Autodesk Inventor part; units mm, degrees
ref_plane "Work Plane1" through (8, 0, 0) normal (0, -0.5, -0.866) x (1, 0, 0)
ref_plane "YZ Plane" through (0, 0, 0) normal (1, 0, 0) x (0, 1, 0)
ref_plane "XZ Plane" through (0, 0, 0) normal (0, 1, 0) x (-1, 0, 0)
sketch "Skizze1" plane through (0, 0, 0) normal (0, 0, 1) x (1, 0, 0)
  line L0 (0.7217, 0) -> (12.1667, 0)
  line L1 (16, 1.4434) -> (16, 2.5)
  line L2 (16, 2.5) -> (0, 2.5)
  line L3 (16, 1.4434) -> (13, 1.4434)
  line L4 (13, 1.4434) -> (12.1667, 0)
  line L5 (0, 1.25) -> (0.7217, 0)
  line L6 (0, -0.5) -> (0, 3)
  line L7 (0, 1.25) -> (0, 2.5)
  point P0 (0, 0)
  dimension "d0" = 3
  dimension "d1" = 60
  dimension "d2" = 5
  dimension "d3" = 2.8868
  dimension "d4" = 16
  dimension "d5" = 60
  dimension "d7" = 2.5
revolve "Körper" add sketch "Skizze1" angle 360 about axis through (0.7217, 0, 0) along (1, 0, 0)
sketch "Skizze2" plane through (16, 0, 0) normal (1, 0, 0) x (0, 0, -1)
  circle A0 centre (0, 0) radius 1.4434
  circle A1 centre (0, 0) radius 2.5
  line L0 (1.4434, 0) -> (0.7217, -1.25)
  line L1 (0.7217, -1.25) -> (-0.7217, -1.25)
  line L2 (-0.7217, -1.25) -> (-1.4434, 0)
  line L3 (-1.4434, 0) -> (-0.7217, 1.25)
  line L4 (-0.7217, 1.25) -> (0.7217, 1.25)
  line L5 (0.7217, 1.25) -> (1.4434, 0)
extrude "Loch" add sketch "Skizze2" against normal blind 3 contours L5 A0 | A0 L0 | L4 A0 | A0 L1 | L3 A0 | A0 L2
chamfer "Fase1" distance 1.25 angle 45 1 edges at (0, -2.5, 0) measured on face at (0, 2.0591, -0.1994)
thread "Gewinde"
chamfer "Fase2" distance 0.4908 angle 45 1 edges at (16, -2.5, 0) measured on face at (11.0832, 2.4676, -0.401)
ref_plane "Work Plane1" through (8, 0, 0) normal (0, -0.5, -0.866) x (1, 0, 0)
equation "\"d0\" = INTI"
equation "\"d2\" = NND"
equation "\"d3\" = 1.1547 * SW"
equation "\"d4\" = NLG"
equation "\"d5\" = 0.5 * ANG"
equation "\"d7\" = SPD"
equation "\"d8\" = INTI"
equation "\"d10\" = -0.5 * SPD + 0.5 * NND"
equation "\"d11\" = FAWI"
equation "\"d33\" = -0.5 * SPD + 0.5 * NND"
equation "\"d14\" = NLG"
equation "\"d12\" = -0.5 * GD1 + 0.5 * NND"
equation "\"d13\" = FAWI"
equation "\"d34\" = -0.5 * GD1 + 0.5 * NND"
equation "\"NND\" = 5"
equation "\"NLG\" = 16"
equation "\"INTI\" = 3"
equation "\"FAWI\" = 45deg"
equation "\"SW\" = 2.5"
equation "\"GD1\" = THREADDIA - 1.2269 * PTC"
equation "\"ANG\" = 120deg"
equation "\"FAWI1\" = 45deg"
equation "\"SPD\" = 2.5"
equation "\"GUL\" = 0.61345 * PTC"
equation "\"TOA\" = 30deg"
equation "\"THREADDIA\" = 5"
equation "\"PTC\" = 0.8"
equation "\"GAL\" = 0.61345 * PTC"
equation "\"E0\" = 1.155 * SW"
properties part number "ISO 4029 - M5 x 16" material "Edelstahl, 440C"
The model under review builds one solid part; all positions refer to its coordinate system, in mm. A direction names the side the tool comes from. Give positions to 0.01 mm unless a question says otherwise; leave off trailing zeros. Order: outer loops, then holes, each group sorted by start corner. A loop starts at its lowest first (then second) coordinate and runs counter-clockwise, first axis right, second up. Notation, with made-up numbers: M 45.5,-38.75 L 52.5,-38.75 A20 cw 52.5,-28.75 Z; hole C 79,0 d4. An arc over 180 degrees is marked long. One line per question, with ' | ' between items. Start each with the question number.
1) Clearance check with flat-ended pins moving along their axes: P1, Ø1, axis at x = 12.5, z = 2, coming from the +Y side; P2, Ø3, axis at x = 13, z = -2, coming from the -Y side; P3, Ø1, axis at x = 4.5, y = -2, coming from the -Z side. State where each tip first meets the part, or that it passes through.
2) For faces 3 (the face through (14.52, 0.63, -1.08)), 4 (the face through (0.596, -0.047, 0.212)), list the 3-axis set-ups (+Z, -Z, +X, -X, +Y, -Y) from which the entire face can be reached by the end or side of a thin tool; tool diameter is ignored.
3) Consider section B-B, the plane x = 3. Give the boundary of the cut face in (y, z), then the cut area to 3 significant figures.
4) Mouldability with a two-part tool opening along Y and no side actions: class faces 1 (the face through (8.28, -0.54, 2.44)), 2 (the face through (14.521, -0.616, -1.088)) as pulls with the +Y half, pulls with the -Y half, needs draft (parallel to the pull), parting line crosses it, or undercut.
5) Consider section A-A, the plane x = 14.75. Give the boundary of the cut face in (y, z), then the cut area to 3 significant figures.
6) Wall thickness on L1, parallel to Y at x = 13.25, z = 1.2; L2, parallel to X at y = 0.2, z = 0.85; L3, parallel to Y at x = 11.25, z = -0.4: over which ranges is each line inside the solid? List them lowest first. Write a range as from..to.
Found:
1) P1: stops at y = 2 | P2: stops at y = -2.45 | P3: stops at z = -2
2) face 3: +X | face 4: -X
3) outline: C 0,0 d5 | area: 19.6 mm²
4) face 1: parting line crosses it | face 2: undercut
5) outline: C 0,0 d5; hole M -1.25,-0.72 L 0,-1.44 L 1.25,-0.72 L 1.25,0.72 L 0,1.44 L -1.25,0.72 Z | area: 14.2 mm²
6) L1: y = -2.19..-0.42, 0.42..2.19 | L2: x = 0.22..12.67 | L3: y = -2.47..2.47
